```python
from build123d import *

# Parameters (mm, degrees)
SKETCH009_R             = 10
SKETCH009_R_2           = 8.15
PAD005_DEPTH            = 30
SKETCH010_R             = 10
PAD006_DEPTH            = 2
SKETCH011_W             = 3
SKETCH011_H             = 13.298698
POCKET004_DEPTH         = 18
SKETCH013_R             = 8.553823
PAD007_DEPTH            = 11
SKETCH012_R             = 1.15
POCKET005_DEPTH         = 21
FILLET002_R             = 1.9
CHAMFER003_SIZE2        = 1.5
CHAMFER003_SIZE         = 5
BODY002_PLACEMENT_ANGLE = 180


with BuildPart() as part:
    # Sketch009 → Pad005 (new body)
    with BuildSketch(Plane.YZ):
        Circle(SKETCH009_R)
        Circle(SKETCH009_R_2, mode=Mode.SUBTRACT)
    extrude(amount=PAD005_DEPTH)

    # Sketch010 (on Face3 of Pad005) → Pad006 (join)
    with BuildSketch(Plane(origin=(0, 0, 0), x_dir=(0, 1, 0), z_dir=(-1, 0, 0))):
        Circle(SKETCH010_R)
    extrude(amount=PAD006_DEPTH)

    # Sketch011 (on Face3 of Pad006) → Pocket004 (cut)
    with BuildSketch(Plane.YZ.offset(30)):
        with Locations((0, 6.649349)):
            Rectangle(SKETCH011_W, SKETCH011_H)
    extrude(amount=-POCKET004_DEPTH, mode=Mode.SUBTRACT)

    # Sketch013 (on Face9 of Pocket004) → Pad007 (join)
    with BuildSketch(Plane.YZ):
        Circle(SKETCH013_R)
    extrude(amount=PAD007_DEPTH)

    # Sketch012 (on DatumPlane) → Pocket005 (cut)
    with BuildSketch(Plane.XY):
        with Locations((4.314017, 0)):
            Circle(SKETCH012_R)
    extrude(amount=POCKET005_DEPTH, mode=Mode.SUBTRACT)

    # Fillet002
    fillet002_edges = [part.edges().sort_by_distance(p)[0] for p in [
        (-2, -10, 0),
    ]]
    fillet(fillet002_edges, radius=FILLET002_R)

    # Chamfer003
    chamfer003_edges = [part.edges().sort_by_distance(p)[0] for p in [
        (30, -6.519202, -7.582875),
        (30, 7.582875, 6.519202),
    ]]
    chamfer003_side = part.faces().sort_by_distance((15, -10, 0))[0]
    chamfer(chamfer003_edges, length=CHAMFER003_SIZE, length2=CHAMFER003_SIZE2, reference=chamfer003_side)


with BuildPart() as part_1:
    # Body002 placement: moved
    add(part.part.moved(Location((282, 0, 14))).rotate(Axis((282, 0, 14), (0, 0, -1)), BODY002_PLACEMENT_ANGLE))


solid = part_1.part
```
For this review, take the finished solid that the model builds, in its own axes (mm). A direction names the side the tool comes from. Coordinates: 2 decimals unless noted, no trailing zeros. Write each loop counter-clockwise with the first axis right and the second up, starting at its lowest first coordinate (ties: lowest second). Pieces come first, ordered by that corner, then holes.
(1) The part is to be moulded in two halves that separate along Z. For faces 5 (the face through (261.633, 1.767, 6.044)), 6 (the face through (278, 0, 14)), 7 (the face through (261, -1.5, 23)), say which applies: +Z half, -Z half, draft (parallel to the pull), parting line (faces both ways), or undercut.
(2) Add section B-B on x = 280.5. Give the boundary of the cut face in (y, z).
(3) Add section C-C on x = 260. Give the boundary of the cut face in (y, z), then the cut area to 3 significant figures.
(4) Tool access review of faces 1 (the face through (276.624, 0.44, 18.931)), 2 (the face through (269.37, -9.54, 11)), 3 (the face through (271, 0, 14)), 4 (the face through (261, 1.5, 23)): name each direction out of +Z, -Z, +X, -X, +Y, -Y from which nothing blocks a thin tool from reaching the whole face with its end or side.
(5) Wall thickness on probe 1 along X at (y, z) = (0, 17.5); probe 2 along Y at (x, z) = (258.75, 14); probe 3 along X at (y, z) = (2, 19.75): over which ranges is each line inside the solid? List them lowest first.
(6) Add section A-A on y = 0. Give the boundary of the cut face in (x, z), then the cut area to 3 significant figures.
(7) For pin 1 Ø1.5 at (x, z) = (262, 23) entering from -Y; pin 2 Ø10 at (x, y) = (258, -3.5) entering from +Z; pin 3 Ø2 at (x, y) = (269.5, -7) entering from -Z, all flat-tipped, find the tip position at first contact; note any pin that passes through.
(8) Add section D-D on x = 256.5. Give the boundary of the cut face in (y, z), then the cut area to 3 significant figures.
Answer sheet:
1. face 5: undercut
1. face 6: +Z half
1. face 7: draft
2. outline: circle Ø20 at (0, 14)
3. outline: (-1.5, 22.01) - (-1.5, 23.89) arc R10 ccw (long way) to (1.5, 23.89) - (1.5, 22.01) arc R8.15 cw (long way) to start
3. area: 99.9 mm2
4. face 1: +Z
4. face 2: +X, -X
4. face 3: -X
4. face 4: +Z, -X
5. probe 1: x = 271 to 276.54, 278.84 to 284
5. probe 2: y = -10 to -8.15, 8.15 to 10
5. probe 3: x = 271 to 284
6. outline: (252, 5.5) - (257, 4) - (282.1, 4) arc R1.9 ccw to (284, 5.9) - (284, 22.1) arc R1.9 ccw to (282.1, 24) - (278.84, 24) - (278.84, 14) - (276.54, 14) - (276.54, 24) - (270, 24) - (270, 22.15) - (271, 22.15) - (271, 5.85) - (252, 5.85) - close
6. area: 269 mm2
7. pin 1: stops at y = -5.65
7. pin 2: stops at z = 23.89
7. pin 3: stops at z = 6
8. outline: (-1.5, 22.01) - (-1.5, 23.74) arc R9.85 ccw (long way) to (1.5, 23.74) - (1.5, 22.01) arc R8.15 cw (long way) to start
8. area: 91.0 mm2
